from build123d import *

# Parameters (mm, degrees)
BOSS_EXTRUDE1_DEPTH = 2
FILLET1_R           = 5
FILLET3_R           = 2
FILLET4_R           = 5


# Read off the part's stored shape, not the designer's step: Boss-Extrude1
with BuildPart() as part:
    # Boss-Extrude1 outline → Boss-Extrude1 (new body)
    with BuildSketch(Plane.XY):
        with BuildLine():
            add(Edge.make_bspline(
                [(50, 0.585067943), (46.302901229, 1.048620246), (37.443381796, 1.911582539), (24.310917963, 2.384537211), (13.949921349, 2.147279936), (6.881664213, 1.770872157), (3.157213928, 1.513128323), (-0.569629629, 1.197220359), (-4.294991328, 0.843416739), (-11.799290896, 0.01694185), (-23.43372993, -1.666844937), (-37.093919746, -4.304130089), (-46.054304433, -6.407794893), (-49.999999999, -7.403419123)],
                knots=[0.392731, 0.392731, 0.392731, 0.392731, 0.4375, 0.5, 0.551677708, 0.562945669, 0.585481591, 0.596749552, 0.608017513, 0.630553434, 0.6875, 0.75, 0.799585435, 0.799585435, 0.799585435, 0.799585435], degree=3))
            Line((50, 0.585067943), (50, -63.46310087))
            Line((50, -63.46310087), (72, -63.46310087))
            Line((72, -63.46310087), (72, 63.46310087))
            Line((72, 63.46310087), (62, 63.46310087))
            Line((62, 63.46310087), (62, -0.17689913))
            Line((62, -0.17689913), (60, -0.17689913))
            Line((60, -0.17689913), (60, 63.46310087))
            Line((60, 63.46310087), (50, 63.46310087))
            Line((50, 63.46310087), (0, 19.391503044))
            Line((0, 19.391503044), (-50, 63.46310087))
            Line((-50, 63.46310087), (-60, 63.46310087))
            Line((-60, 63.46310087), (-60, -0.17689913))
            Line((-60, -0.17689913), (-62, -0.17689913))
            Line((-62, -0.17689913), (-62, 63.46310087))
            Line((-62, 63.46310087), (-72, 63.46310087))
            Line((-72, 63.46310087), (-72, -63.46310087))
            Line((-72, -63.46310087), (-50, -63.46310087))
            Line((-50, -63.46310087), (-49.999999999, -7.403419123))
        make_face()
        with BuildLine():
            add(Edge.make_bspline(
                [(-5.349354195, 10.7764699), (-6.473284635, 10.660224491), (-12.934279192, 9.954218876), (-24.646320739, 8.284783337), (-38.353198567, 5.637906199), (-46.754684535, 3.697054478), (-49.999999999, 2.901338723)],
                knots=[0.611854507, 0.611854507, 0.611854507, 0.611854507, 0.625, 0.6875, 0.75, 0.789622747, 0.789622747, 0.789622747, 0.789622747], degree=3))
            Line((-49.999999999, 2.901338723), (-50, 50.132975987))
            Line((-50, 50.132975987), (-5.349354195, 10.7764699))
        make_face(mode=Mode.SUBTRACT)
        with BuildLine():
            Line((50, 50.132975987), (50, 10.659702462))
            add(Edge.make_bspline(
                [(50, 10.659702462), (46.536536843, 11.073334631), (37.671385716, 11.912189244), (23.444000892, 12.423604272), (12.413305008, 12.108752618), (6.751894701, 11.770134287), (6.456063808, 11.751959115)],
                knots=[0.397516142, 0.397516142, 0.397516142, 0.397516142, 0.4375, 0.5, 0.5625, 0.565946061, 0.565946061, 0.565946061, 0.565946061], degree=3))
            Line((6.456063808, 11.751959115), (50, 50.132975987))
        make_face(mode=Mode.SUBTRACT)
    extrude(amount=BOSS_EXTRUDE1_DEPTH)

    # Fillet1
    fillet1_edges = [part.edges().sort_by_distance(p)[0] for p in [
        (-72, -63.46310087, 1),
        (-72, 63.46310087, 1),
        (-50, 63.46310087, 1),
        (50, 63.46310087, 1),
        (72, 63.46310087, 1),
        (50, 0.585067943, 1),
        (72, -63.46310087, 1),
        (50, -63.46310087, 1),
        (-50, -63.46310087, 1),
        (-49.999999999, -7.403419123, 1),
        (0, 19.391503044, 1),
    ]]
    fillet(fillet1_edges, radius=FILLET1_R)

    # Fillet3
    fillet3_edges = [part.edges().sort_by_distance(p)[0] for p in [
        (-62, 63.46310087, 1),
        (-60, 63.46310087, 1),
        (60, 63.46310087, 1),
        (62, 63.46310087, 1),
    ]]
    fillet(fillet3_edges, radius=FILLET3_R)

    # Fillet4
    fillet4_edges = [part.edges().sort_by_distance(p)[0] for p in [
        (50, 50.132975987, 1),
        (6.456063808, 11.751959115, 1),
        (50, 10.659702462, 1),
        (-50, 50.132975987, 1),
        (-49.999999999, 2.901338723, 1),
        (-5.349354195, 10.7764699, 1),
    ]]
    fillet(fillet4_edges, radius=FILLET4_R)


solid = part.part
The listing builds one solid part. Answer for the finished solid, in the listing's coordinates (mm). A direction names the side the tool comes from. Coordinates: 2 decimals unless noted, no trailing zeros. Loops run counter-clockwise (first coordinate to the right, second up) from the corner with the lowest first, then second, coordinate; pieces in that order, holes last.
1) Find section C-C on y = 34. Write down the section's boundary in (x, z), then the cut area to 3 significant figures.
2) Find section B-B on y = 50. Write down the section's boundary in (x, z), then the cut area to 3 significant figures.
3) A flat-ended cylindrical pin translates along its axis: pin 1 Ø2 at (x, y) = (-27.5, 44.5) entering from +Z. Find the tip coordinate at first contact, or state that the pin passes through.
4) Find section A-A on y = -21. Write down the section's boundary in (x, z).
5) Determine the mould class of faces 1 (the face through (70.574, 61.96, 1.014)), 2 (the face through (-51.426, -61.96, 1.014)), 3 (the face through (1, 15, 0)) for opening direction X: pulls with the +X half, pulls with the -X half, needs draft (parallel to the pull), parting line crosses it, or undercut.
6) Find section D-D on z = 1.4. Give the number of separate pieces and of enclosed holes in the cut face, then the cut area to 3 significant figures.
7) A tool of negligible diameter and unlimited length cuts with its end or side. For faces 4 (the face through (26.26, 42.54, 0.99)), 5 (the face through (70.496, -62.037, 1.014)), 6 (the face through (47.1, 43.6, 1)), 7 (the face through (51.426, -61.96, 1.014)), from which of +Z, -Z, +X, -X, +Y, -Y can it reach the whole face along a straight path? Write none if from no direction.
8) Find the intervals of material crossed by L1, parallel to X at y = 4, z = 1.95; L2, parallel to X at y = 35, z = 0.95; L3, parallel to X at y = 46, z = 1.4, in increasing order.
Values:
1. outline: (-72, 0) - (-62, 0) - (-62, 2) - (-72, 2) - close; (-60, 0) - (-50, 0) - (-50, 2) - (-60, 2) - close; (-31.7, 0) - (-16.57, 0) - (-16.57, 2) - (-31.7, 2) - close; (16.57, 0) - (31.7, 0) - (31.7, 2) - (16.57, 2) - close; (50, 0) - (60, 0) - (60, 2) - (50, 2) - close; (62, 0) - (72, 0) - (72, 2) - (62, 2) - close
1. area: 140 mm2
2. outline: (-72, 0) - (-62, 0) - (-62, 2) - (-72, 2) - close; (-60, 0) - (-34.73, 0) - (-34.73, 2) - (-60, 2) - close; (34.73, 0) - (60, 0) - (60, 2) - (34.73, 2) - close; (62, 0) - (72, 0) - (72, 2) - (62, 2) - close
2. area: 141 mm2
3. pin 1: stops at z = 2
4. outline: (-72, 0) - (-50, 0) - (-50, 2) - (-72, 2) - close; (50, 0) - (72, 0) - (72, 2) - (50, 2) - close
5. face 1: pulls with the +X half
5. face 2: undercut
5. face 3: needs draft
6. separate pieces: 1
6. enclosed holes: 2
6. area: 7,750 mm2
7. face 4: +Z, -Z, +Y
7. face 5: +Z, -Z, +X, -Y
7. face 6: +Z, -Z
7. face 7: +Z, -Z, -Y
8. L1: x = -72 to -62, -60 to 60, 62 to 72
8. L2: x = -72 to -62, -60 to -50, -32.83 to -17.71, 17.71 to 32.83, 50 to 60, 62 to 72
8. L3: x = -72 to -62, -60 to -30.19, 30.19 to 60, 62 to 72
